from build123d import *

# Parameters (mm, degrees)
BOSS_EXTRUDE1_DEPTH = 78
SKETCH2_W           = 30
SKETCH2_H           = 35
BOSS_EXTRUDE2_DEPTH = 5


with BuildPart() as part:
    # Sketch1 → Boss-Extrude1 (new body)
    with BuildSketch(Plane(origin=(0, 0, 0), x_dir=(1, 0, 0), z_dir=(0, 1, 0))):
        with BuildLine():
            Line((-6.024549776, 13.633018741), (7.608468966, 0))
            Line((7.608468966, 0), (-6.024549776, -13.633018741))
            ThreePointArc((-6.024549776, -13.633018741), (-9.814642123, -13.633018741), (-9.814642123, -9.842926394))
            Line((-9.814642123, -9.842926394), (-0.706968119, -0.735252391))
            ThreePointArc((-0.706968119, -0.735252391), (1.02, 0), (-0.706968119, 0.735252391))
            Line((-0.706968119, 0.735252391), (-9.814642123, 9.842926394))
            ThreePointArc((-9.814642123, 9.842926394), (-9.814642123, 13.633018741), (-6.024549776, 13.633018741))
        make_face()
    extrude(amount=BOSS_EXTRUDE1_DEPTH)

    # Sketch2 → Boss-Extrude2 (add)
    with BuildSketch(Plane(origin=(0, 78, 0), x_dir=(1, 0, 0), z_dir=(0, 1, 0))):
        with Locations((-2.479307664, -0.975058093)):
            Rectangle(SKETCH2_W, SKETCH2_H)
    extrude(amount=BOSS_EXTRUDE2_DEPTH)


solid = part.part
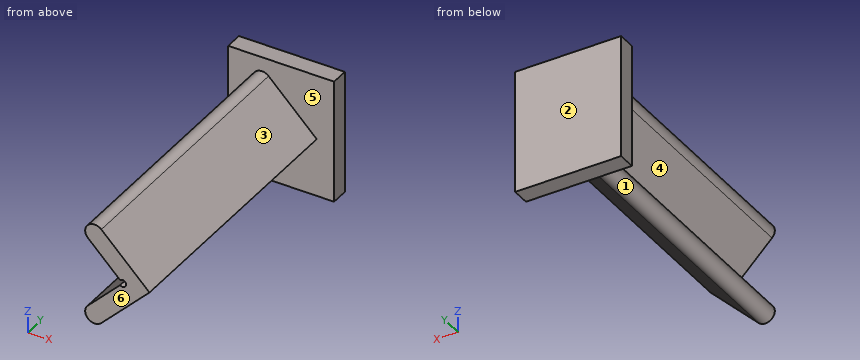
Build history of the part. All positions in model axes, mm. Face numbers are marked on the shaded views. A direction names the side the tool comes from. Give positions to 0.01 mm unless a question says otherwise; leave off trailing zeros. Order: outer loops, then holes, each group sorted by start corner. A loop starts at its lowest first (then second) coordinate and runs counter-clockwise, first axis right, second up. Notation, with made-up numbers: M 69,74.25 L 92,74.25 A21 cw 92,81.25 Z; hole C -21.5,30.5 d8. An arc over 180 degrees is marked long. Put each result on its own line as item: value.
Item 1: Cut at B-B on x = -5. Write the cut outline in (y, z), then the cut area to 3 significant figures.
Results are:
outline: M 0,-12.61 L 78,-12.61 L 78,-16.52 L 83,-16.52 L 83,18.48 L 78,18.48 L 78,12.61 L 0,12.61 L 0,5.03 L 78,5.03 L 78,-5.03 L 0,-5.03 Z
area: 1,360 mm2
Item 2: Cut at C-C on z = -6.5. Write the cut outline in (x, y), then the cut area to 3 significant figures.
Results are:
outline: M -17.48,78 L -6.47,78 L -6.47,0 L 1.11,0 L 1.11,78 L 12.52,78 L 12.52,83 L -17.48,83 Z
area: 741 mm2
Item 3: Drop flat-ended pins along their axis: pin 1 Ø8 at (x, y) = (-12.5, 46.5) entering from +Z; pin 2 Ø1.5 at (x, y) = (-6.5, 51.5) entering from +Z; pin 3 Ø5 at (y, z) = (72.5, 6.5) entering from +X. Give the stop position or say it passes through.
Results are:
pin 1: z = 14.35
pin 2: z = 14.33
pin 3: x = 3.61
Item 4: Pull direction Z, two halves, no side cores. Call the marked faces 1, 2 and 3: +Z half, -Z half, draft (parallel to the pull), parting line (faces both ways), or undercut.
Results are:
face 1: undercut
face 2: draft
face 3: +Z half
Item 5: Which spindle directions (+Z, -Z, +X, -X, +Y, -Y) get a long thin tool onto all of the face, cutting with end or side? Do the marked faces 4, 5 and 6. Say none if no direction does.
Results are:
face 4: -X, -Y
face 5: -Y
face 6: +Z, -Z, +X, -X, -Y
Item 6: Cut at D-D on x = 5.5. Write the cut outline in (y, z), then the cut area to 3 significant figures.
Results are:
outline: M 0,-2.11 L 78,-2.11 L 78,-16.52 L 83,-16.52 L 83,18.48 L 78,18.48 L 78,2.11 L 0,2.11 Z
area: 504 mm2
Item 7: Wall check: probe 1 along Y at (x, z) = (1, -7); probe 2 along Z at (x, y) = (0, 25.5); probe 3 along X at (y, z) = (19, 0). Give the ranges that are in metal, low to high.
Results are:
probe 1: 78 to 83
probe 2: -7.61 to -1.02, 1.02 to 7.61
probe 3: 1.02 to 7.61
Item 8: Cut at A-A on y = 76. Write the cut outline in (x, z).
Results are:
outline: M -9.81,-9.84 A2.68 ccw -6.02,-13.63 L 7.61,0 L -6.02,13.63 A2.68 ccw -9.81,9.84 L -0.71,0.74 A1.02 cw long -0.71,-0.74 Z
